Source: CAD feature listing. Evaluate the final solid. Frame: model axes, mm. A direction names the side the tool comes from. Coordinates: 2 decimals unless noted, no trailing zeros. Write each loop counter-clockwise with the first axis right and the second up, starting at its lowest first coordinate (ties: lowest second). Pieces come first, ordered by that corner, then holes. Notation, with made-up numbers: M 23.25,-12.75 L 55.25,-12.75 A30 cw 55.25,23.25 Z; hole C -24,54.25 d5. An arc over 180 degrees is marked long. Write item = value, one per line. Start each with the question number.
1. Section query D-D (y = -1.55). Output: boundary loops of the cut face in (x, z), then the cut area to 3 significant figures.
2. Section query B-B (y = 0.05). Output: boundary loops of the cut face in (x, z).
3. Line query: line 1 along Z through (x, y) = (1.5, 0.2); line 2 along Y through (x, z) = (0.25, -1.4). Output: solid intervals per line, ascending.
4. Pin query (flat end, axial travel): pin 1 Ø1.5 at (y, z) = (-0.5, -1.5) entering from +X. Return the tip coordinate at first contact, or that it passes through.
5. Section query A-A (x = 0.5). Output: boundary loops of the cut face in (y, z), then the cut area to 3 significant figures.
6. Section query C-C (z = -1.5). Output: boundary loops of the cut face in (x, y).
7. Access query for faces 1 (the face through (0, 1.25, -1)), 2 (the face through (0, -1.25, -1)), 3 (the face through (-1.25, 0, -1)). Directions: +Z, -Z, +X, -X, +Y, -Y. A direction counts if a zero-diameter tool reaches every point of the face in a straight line with its end or side. Return the directions, or none.
```python
from build123d import *

# Parameters (mm, degrees)
SKETCH1_W           = 9.2
SKETCH1_H           = 3.6
BOSS_EXTRUDE1_DEPTH = 3
SKETCH2_W           = 2.5
SKETCH2_H           = 2.5
BOSS_EXTRUDE2_DEPTH = 2


with BuildPart() as part:
    # Sketch1 → Boss-Extrude1 (new body)
    with BuildSketch(Plane.XY):
        Rectangle(SKETCH1_W, SKETCH1_H)
    extrude(amount=BOSS_EXTRUDE1_DEPTH)

    # Sketch2 → Boss-Extrude2 (add)
    with BuildSketch(Plane(origin=(0, 0, 0), x_dir=(-1, 0, 0), z_dir=(0, 0, -1))):
        Rectangle(SKETCH2_W, SKETCH2_H)
    extrude(amount=BOSS_EXTRUDE2_DEPTH)


solid = part.part
```
Results are:
q1.outline = M -4.6,0 L 4.6,0 L 4.6,3 L -4.6,3 Z
q1.area = 27.6 mm^2
q2.outline = M -4.6,0 L -1.25,0 L -1.25,-2 L 1.25,-2 L 1.25,0 L 4.6,0 L 4.6,3 L -4.6,3 Z
q3.line_1 = 0 to 3
q3.line_2 = -1.25 to 1.25
q4.pin_1 = 1.25
q5.outline = M -1.8,0 L -1.25,0 L -1.25,-2 L 1.25,-2 L 1.25,0 L 1.8,0 L 1.8,3 L -1.8,3 Z
q5.area = 15.8 mm^2
q6.outline = M -1.25,-1.25 L 1.25,-1.25 L 1.25,1.25 L -1.25,1.25 Z
q7.face_1 = -Z, +X, -X, +Y
q7.face_2 = -Z, +X, -X, -Y
q7.face_3 = -Z, -X, +Y, -Y
